Work out the finished part from the listing and answer in its coordinate system (mm). A direction names the side the tool comes from. Coordinates: 2 decimals unless noted, no trailing zeros. Order: outer loops, then holes, each group sorted by start corner. A loop starts at its lowest first (then second) coordinate and runs counter-clockwise, first axis right, second up.
```python
from build123d import *

# Parameters (mm, degrees)
F0_R     = 5.08
F0_R_2   = 5.3975
F1_DEPTH = 6.35


# Not quite as in the source:
# - a feature names something its author has since deleted; it is built from what else it names


with BuildPart() as f1:
    # F0 (on Front) → F1 (new body)
    with BuildSketch(Plane.XZ):
        with BuildLine():
            Line((34.9250002354, -44.45), (57.1500004709, -44.45))
            Line((57.1500004709, -44.45), (63.5, -44.45))
            Line((63.5, -44.45), (63.5, -12.7))
            Line((63.5, -12.7), (57.1500004709, -12.7))
            Line((57.1500004709, -12.7), (57.1500004709, -1.4605))
            Line((57.1500004709, -1.4605), (52.7050002354, -1.4605))
            Line((52.7050002354, -1.4605), (52.7050002354, -2.69367))
            Line((52.7050002354, -2.69367), (50.1650002354, -2.69367))
            Line((50.1650002354, -2.69367), (50.1650002354, -1.4605))
            Line((50.1650002354, -1.4605), (45.72, -1.4605))
            Line((45.72, -1.4605), (45.72, 1.4605))
            Line((45.72, 1.4605), (50.1650002354, 1.4605))
            Line((50.1650002354, 1.4605), (50.1650002354, 2.69367))
            Line((50.1650002354, 2.69367), (52.7050002354, 2.69367))
            Line((52.7050002354, 2.69367), (52.7050002354, 1.4605))
            Line((52.7050002354, 1.4605), (57.1500004709, 1.4605))
            Line((57.1500004709, 1.4605), (57.1500004709, 12.7))
            Line((57.1500004709, 12.7), (63.5, 12.7))
            Line((63.5, 12.7), (63.5, 44.45))
            Line((63.5, 44.45), (57.1500004709, 44.45))
            Line((57.1500004709, 44.45), (34.9250002354, 44.45))
            Line((34.9250002354, 44.45), (34.9250002354, 35.306))
            Line((34.9250002354, 35.306), (42.5450002354, 35.306))
            Line((42.5450002354, 35.306), (42.5450002354, 21.844))
            Line((42.5450002354, 21.844), (34.9250002354, 21.844))
            Line((34.9250002354, 21.844), (34.9250002354, -12.7))
            Line((34.9250002354, -12.7), (45.7200002354, -12.7))
            ThreePointArc((45.7200002354, -12.7), (47.5160514597, -13.4439487758), (48.2600002354, -15.24))
            Line((48.2600002354, -15.24), (48.2600002354, -24.5090161092))
            ThreePointArc((48.2600002354, -24.5090161092), (48.1168161661, -25.3497737405), (47.7034070114, -26.09574153))
            Line((47.7034070114, -26.09574153), (43.9426198988, -30.7967254208))
            ThreePointArc((43.9426198988, -30.7967254208), (43.0595124983, -31.4993102202), (41.9592131228, -31.75))
            Line((41.9592131228, -31.75), (34.9250002354, -31.75))
            Line((34.9250002354, -31.75), (34.9250002354, -44.45))
        make_face()
        with BuildLine():
            Line((12.7, -44.45), (34.9250002354, -44.45))
            Line((34.9250002354, -44.45), (34.9250002354, -31.75))
            Line((34.9250002354, -31.75), (27.8907873481, -31.75))
            ThreePointArc((27.8907873481, -31.75), (26.7904879726, -31.4993102202), (25.9073805721, -30.7967254208))
            Line((25.9073805721, -30.7967254208), (22.1465934595, -26.09574153))
            ThreePointArc((22.1465934595, -26.09574153), (21.7331843048, -25.3497737405), (21.5900002354, -24.5090161092))
            Line((21.5900002354, -24.5090161092), (21.5900002354, -15.24))
            ThreePointArc((21.5900002354, -15.24), (22.3339490112, -13.4439487758), (24.1300002354, -12.7))
            Line((24.1300002354, -12.7), (34.9250002354, -12.7))
            Line((34.9250002354, -12.7), (34.9250002354, 21.844))
            Line((34.9250002354, 21.844), (27.3050002354, 21.844))
            Line((27.3050002354, 21.844), (27.3050002354, 35.306))
            Line((27.3050002354, 35.306), (34.9250002354, 35.306))
            Line((34.9250002354, 35.306), (34.9250002354, 44.45))
            Line((34.9250002354, 44.45), (12.7, 44.45))
            Line((12.7, 44.45), (12.7, 38.1000004709))
            Line((12.7, 38.1000004709), (1.4605, 38.1000004709))
            Line((1.4605, 38.1000004709), (1.4605, 33.6550002354))
            Line((1.4605, 33.6550002354), (2.69367, 33.6550002354))
            Line((2.69367, 33.6550002354), (2.69367, 31.1150002354))
            Line((2.69367, 31.1150002354), (1.4605, 31.1150002354))
            Line((1.4605, 31.1150002354), (1.4605, 26.67))
            Line((1.4605, 26.67), (-1.4605, 26.67))
            Line((-1.4605, 26.67), (-1.4605, 31.1150002354))
            Line((-1.4605, 31.1150002354), (-2.69367, 31.1150002354))
            Line((-2.69367, 31.1150002354), (-2.69367, 33.6550002354))
            Line((-2.69367, 33.6550002354), (-1.4605, 33.6550002354))
            Line((-1.4605, 33.6550002354), (-1.4605, 38.1000004709))
            Line((-1.4605, 38.1000004709), (-12.7, 38.1000004709))
            Line((-12.7, 38.1000004709), (-12.7, 44.45))
            Line((-12.7, 44.45), (-57.1500004709, 44.45))
            Line((-57.1500004709, 44.45), (-63.5, 44.45))
            Line((-63.5, 44.45), (-63.5, 12.7))
            Line((-63.5, 12.7), (-57.1500004709, 12.7))
            Line((-57.1500004709, 12.7), (-57.1500004709, 1.4605))
            Line((-57.1500004709, 1.4605), (-52.7050002354, 1.4605))
            Line((-52.7050002354, 1.4605), (-52.7050002354, 2.69367))
            Line((-52.7050002354, 2.69367), (-50.1650002354, 2.69367))
            Line((-50.1650002354, 2.69367), (-50.1650002354, 1.4605))
            Line((-50.1650002354, 1.4605), (-45.72, 1.4605))
            Line((-45.72, 1.4605), (-45.72, -1.4605))
            Line((-45.72, -1.4605), (-50.1650002354, -1.4605))
            Line((-50.1650002354, -1.4605), (-50.1650002354, -2.69367))
            Line((-50.1650002354, -2.69367), (-52.7050002354, -2.69367))
            Line((-52.7050002354, -2.69367), (-52.7050002354, -1.4605))
            Line((-52.7050002354, -1.4605), (-57.1500004709, -1.4605))
            Line((-57.1500004709, -1.4605), (-57.1500004709, -2.69367))
            Line((-57.1500004709, -2.69367), (-57.1500004709, -12.7))
            Line((-57.1500004709, -12.7), (-63.5, -12.7))
            Line((-63.5, -12.7), (-63.5, -44.45))
            Line((-63.5, -44.45), (-57.1500004709, -44.45))
            Line((-57.1500004709, -44.45), (-12.7, -44.45))
            Line((-12.7, -44.45), (-12.7, -38.1000004709))
            Line((-12.7, -38.1000004709), (-1.4605, -38.1000004709))
            Line((-1.4605, -38.1000004709), (-1.4605, -33.6550002354))
            Line((-1.4605, -33.6550002354), (-2.69367, -33.6550002354))
            Line((-2.69367, -33.6550002354), (-2.69367, -31.1150002354))
            Line((-2.69367, -31.1150002354), (-1.4605, -31.1150002354))
            Line((-1.4605, -31.1150002354), (-1.4605, -26.67))
            Line((-1.4605, -26.67), (1.4605, -26.67))
            Line((1.4605, -26.67), (1.4605, -31.1150002354))
            Line((1.4605, -31.1150002354), (2.69367, -31.1150002354))
            Line((2.69367, -31.1150002354), (2.69367, -33.6550002354))
            Line((2.69367, -33.6550002354), (1.4605, -33.6550002354))
            Line((1.4605, -33.6550002354), (1.4605, -38.1000004709))
            Line((1.4605, -38.1000004709), (12.7, -38.1000004709))
            Line((12.7, -38.1000004709), (12.7, -44.45))
        make_face()
        with Locations((-34.9250002354, -19.8745080546)):
            Circle(F0_R, mode=Mode.SUBTRACT)
        with Locations((-34.9250002354, 28.575)):
            Circle(F0_R_2, mode=Mode.SUBTRACT)
    extrude(amount=F1_DEPTH)


solid = f1.part
```
1. The part is cut by section D-D (y = -3.75). Count the separate pieces of the cut face and the enclosed holes in it, plus the area to 3 significant figures.
2. Consider probe 1 along X at (y, z) = (-1.5, -19.5); probe 2 along X at (y, z) = (-0.75, 29) (1 decimal); probe 3 along Z at (x, y) = (-50.5, -0.75). Determine where each line is inside the solid, lowest interval first.
3. Flat-ended cylindrical pins translate along their axes: pin 1 (1.5 mm diameter, centred on x = 2.5, y = -5.5, fed in from +Z); pin 2 (0.6 mm diameter, centred on y = -3.5, z = -2, fed in from -X); pin 3 (3 mm diameter, centred on y = -3.5, z = 5, fed in from +X); pin 4 (6.5 mm diameter, centred on x = -34.925, z = 28.575, fed in from +Y). Find the tip coordinate at first contact, or state that the pin passes through.
4. The part is cut by section A-A (x = 36). Determine the outline of the cut face in (y, z).
5. The part is cut by section B-B (z = 25). Determine the outline of the cut face in (x, y) (3 decimals), plus the area to 3 significant figures.
6. The part is cut by section C-C (x = -4.5). Determine the outline of the cut face in (y, z), plus the area to 3 significant figures.
7. For faces 1 (the flat face through (-1.46, -3, 29)), 2 (the flat face through (-55, -3, -1.46)), 3 (the flat face through (21.59, -3, -20)), determine the directions among +Z, -Z, +X, -X, +Y, -Y from which every point of the face is accessible in a straight line to the end or side of a thin tool.
8. The mould has two halves that part along X. Classify faces 4 (the flat face through (57.15, -3, -7)), 5 (the flat face through (-45.72, -3, 0)), 6 (the flat face through (-2.694, -3, 32)): released by +X, released by -X, zero draft, split by the parting line, or undercut.
Worked out:
1. separate pieces: 1
1. enclosed holes: 4
1. area: 9,640 mm2
2. probe 1: x = -63.5 to -39.99, -29.86 to 21.59, 48.26 to 63.5
2. probe 2: x = -63.5 to -40.3, -29.5 to -1.5, 1.5 to 27.3, 42.5 to 63.5
2. probe 3: z = -44.45 to -2.69, 2.69 to 44.45
3. pin 1: stops at z = 38.1
3. pin 2: stops at x = -57.15
3. pin 3: stops at x = 57.15
3. pin 4: passes through
4. outline: (-6.35, -44.45) - (0, -44.45) - (0, -31.75) - (-6.35, -31.75) - close; (-6.35, -12.7) - (0, -12.7) - (0, 21.84) - (-6.35, 21.84) - close; (-6.35, 35.31) - (0, 35.31) - (0, 44.45) - (-6.35, 44.45) - close
5. outline: (-63.5, -6.35) - (-38.969, -6.35) - (-38.969, 0) - (-63.5, 0) - close; (-30.881, -6.35) - (27.305, -6.35) - (27.305, 0) - (-30.881, 0) - close; (42.545, -6.35) - (63.5, -6.35) - (63.5, 0) - (42.545, 0) - close
5. area: 658 mm2
6. outline: (-6.35, -38.1) - (0, -38.1) - (0, 38.1) - (-6.35, 38.1) - close
6. area: 484 mm2
7. face 1: +Z, +Y, -Y
7. face 2: -X, +Y, -Y
7. face 3: +Y, -Y
8. face 4: released by +X
8. face 5: released by -X
8. face 6: undercut
